Could you check a few things on this model? Use its own coordinates, in mm. Face numbers are marked on the shaded views. A direction names the side the tool comes from. Coordinates: 2 decimals unless noted, no trailing zeros. Loops run counter-clockwise (first coordinate to the right, second up) from the corner with the lowest first, then second, coordinate; pieces in that order, holes last.
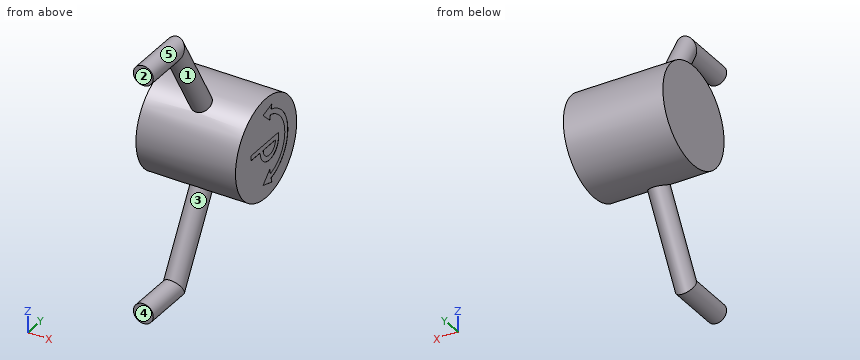
from build123d import *

# Parameters (mm, degrees)
SKETCH1_R           = 50
BOSS_EXTRUDE1_DEPTH = 50
SWEEP1_PROFILE_R    = 10
CUT_EXTRUDE1_DEPTH  = 0.1


with BuildPart() as part:
    # Sketch1 → Boss-Extrude1 (new, symmetric)
    with BuildSketch(Plane(origin=(0, 0, 0), x_dir=(0, 0, -1), z_dir=(1, 0, 0))):
        Circle(SKETCH1_R)
    extrude(amount=BOSS_EXTRUDE1_DEPTH, both=True)

    # Sweep1: sweep along a path in Sketch2
    with BuildLine(Plane(origin=(0, 0, 0), x_dir=(0, 0, -1), z_dir=(1, 0, 0))) as sweep1_path:
        Line((0, 0), (-120, -69.282032303))
        Line((-120, -69.282032303), (-120, -119.282032303))
    # Sweep1 profile (on start of the path) → Sweep1 (sweep)
    with BuildSketch(Plane(origin=(0, 0, 0), x_dir=(0, 0.866025403784438, 0.5000000000000012), z_dir=(0, -0.5000000000000012, 0.866025403784438))):
        Circle(SWEEP1_PROFILE_R)
    sweep1 = sweep(path=sweep1_path.line, transition=Transition.RIGHT)

    # Mirror1: Sweep1 across plane
    add(sweep1.mirror(Plane.XY))

    # Sketch13 → Cut-Extrude1 (cut)
    # profile 1 of 2: a face of its own
    with BuildSketch(Plane(origin=(50, 0, 0), x_dir=(0, 0, -1), z_dir=(1, 0, 0))):
        with BuildLine():
            Line((-34.63127072, 8.321411489), (-39.492891462, 9.489591167))
            Line((-39.492891462, 9.489591167), (-35.235480182, -4.893539549))
            Line((-35.235480182, -4.893539549), (-24.908029236, 5.985052132))
            Line((-24.908029236, 5.985052132), (-29.769649978, 7.15323181))
            ThreePointArc((-29.769649978, 7.15323181), (0, 30.61700157), (29.769649978, 7.15323181))
            Line((29.769649978, 7.15323181), (24.908029236, 5.985052132))
            Line((24.908029236, 5.985052132), (35.235480182, -4.893539549))
            Line((35.235480182, -4.893539549), (39.492891462, 9.489591167))
            Line((39.492891462, 9.489591167), (34.63127072, 8.321411489))
            ThreePointArc((34.63127072, 8.321411489), (0, 35.61700157), (-34.63127072, 8.321411489))
        make_face()
    # profile 2 of 2: a face of its own
    with BuildSketch(Plane(origin=(50, 0, 0), x_dir=(0, 0, -1), z_dir=(1, 0, 0))):
        with BuildLine():
            Line((-5, 20.386275511), (-5, -24.532723242))
            ThreePointArc((-5, -24.532723242), (-2.499671961, -24.552974882), (0, -24.613724489))
            Line((0, -24.613724489), (0, -9.613724489))
            ThreePointArc((0, -9.613724489), (15, 5.386275511), (0, 20.386275511))
            Line((0, 20.386275511), (-5, 20.386275511))
        make_face()
        with BuildLine():
            Line((0, 15.386275511), (0, -4.613724489))
            ThreePointArc((0, -4.613724489), (10, 5.386275511), (0, 15.386275511))
        make_face(mode=Mode.SUBTRACT)
    extrude(amount=-CUT_EXTRUDE1_DEPTH, mode=Mode.SUBTRACT)


solid = part.part
(1) Imagine slicing it at B-B, the plane z = -6. Write out the boundary of the cut face in (x, y).
Answers:
outline: (-50, -49.64) - (50, -49.64) - (50, -8.36) - (49.9, -8.36) - (49.9, -2.61) - (50, -2.61) - (50, 13.39) - (49.9, 13.39) - (49.9, 19.13) - (50, 19.13) - (50, 30.02) - (49.9, 30.02) - (49.9, 35.11) - (50, 35.11) - (50, 49.64) - (-50, 49.64) - close
(2) Imagine slicing it at A-A, the plane y = -92. Write out the boundary of the cut face in (x, z), and give its area (3 significant figures).
Answers:
outline: circle Ø20 at (0, -120); circle Ø20 at (0, 120)
area: 628 mm2
(3) Imagine slicing it at C-C, the plane x = 0. Write out the boundary of the cut face in (y, z), and give its area (3 significant figures).
Answers:
outline: (-119.28, -130) - (-63.51, -130) - (-15.83, -47.43) arc R50 ccw (long way) to (-15.83, 47.43) - (-63.51, 130) - (-119.28, 130) - (-119.28, 110) - (-75.06, 110) - (-33.16, 37.43) arc R50 ccw to (-33.16, -37.43) - (-75.06, -110) - (-119.28, -110) - close
area: 13,400 mm2
(4) We'd pull the mould along Z, two halves only. Please class the marked faces 1, 2 and 3: +Z half, -Z half, draft (parallel to the pull), parting line (faces both ways), or undercut.
Answers:
face 1: undercut
face 2: draft
face 3: undercut
(5) Which directions (+Z, -Z, +X, -X, +Y, -Y) give clear straight access to the entire face, cutting with the end or side of a thin tool? Please do the marked faces 4 and 5.
Answers:
face 4: +Z, -Z, +X, -X, -Y
face 5: -Y
(6) I need wall thicknesses on probe 1 along Z at (x, y) = (-28.5, 15); probe 2 along Z at (x, y) = (30, 7.5); probe 3 along Y at (x, z) = (-7.5, 40). Which ranges of each line are inside material? Lowest first, please.
Answers:
probe 1: z = -47.7 to 47.7
probe 2: z = -49.43 to 49.43
probe 3: y = -30.73 to 30
(7) For pin 1 (12 mm diameter, centred on x = -24.5, y = -26.5, fed in from -Z); pin 2 (8 mm diameter, centred on x = -24, z = 33.5, fed in from -Y); pin 3 (8 mm diameter, centred on x = -30.5, z = -34.5, fed in from -Y), each with a flat end and sliding along its axis, tell me the tip position at first contact or that it passes through.
Answers:
pin 1: stops at z = -45.6
pin 2: stops at y = -40.37
pin 3: stops at y = -39.62
(8) Imagine slicing it at D-D, the plane y = 0. Write out the boundary of the cut face in (x, z).
Answers:
outline: (-50, -50) - (50, -50) - (50, -36.68) - (49.9, -36.68) - (49.9, -30.59) - (50, -30.59) - (50, -14) - (49.9, -14) - (49.9, -8.43) - (50, -8.43) - (50, 0) - (49.9, 0) - (49.9, 5) - (50, 5) - (50, 30.59) - (49.9, 30.59) - (49.9, 36.68) - (50, 36.68) - (50, 50) - (-50, 50) - close
